Source: CAD feature listing. Evaluate the final solid. Frame: model axes, mm. Face numbers are marked on the shaded views. A direction names the side the tool comes from. Coordinates: 2 decimals unless noted, no trailing zeros. Order: outer loops, then holes, each group sorted by start corner. A loop starts at its lowest first (then second) coordinate and runs counter-clockwise, first axis right, second up.
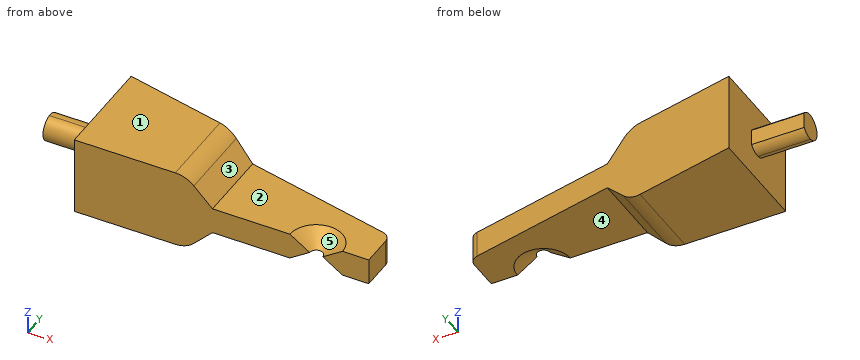
Autodesk Inventor part; units mm, degrees
ref_plane "Work Plane2" through (15.7073, 3, 0) normal (-1, 0, 0) x (0, 0, -1)
ref_plane "Work Plane5" through (10.5053, 0, 0) normal (0, 0, 1) x (1, 0, 0)
ref_plane "YZ Plane" through (0, 0, 0) normal (1, 0, 0) x (0, 1, 0)
sketch "Sketch1" plane through (0, 0, 0) normal (0, 0, 1) x (1, 0, 0)
  line L0 (0, 8) -> (22.3923, 3)
  line L1 (22.3923, 0) -> (22.3923, 3)
  line L2 (0, 0) -> (22.3923, 0)
  line L3 (0, 8) -> (0, 0)
  dimension "d5" = 3
  dimension "d7" = 8
  dimension "d59" = 22.3923
extrude "Extrusion1" add sketch "Sketch1" along normal mid plane 6
sketch "Sketch2" plane through (0, 0, 3) normal (-1, 0, 0) x (0, 0, 1)
  line L0 (-6, 0) -> (-6, 8)
  line L1 (0, 3) -> (0, 8)
  line L2 (-6, 0) -> (0, 8)
  line L3 (-6, 8) -> (0, 8)
  line L4 (0, 8) -> (0, 0)
  line L5 (-6, 8) -> (0, 0)
  arc A0 (-3.995, 3.9001) -> (-2.005, 3.9001) centre (-3, 4) ccw
  line L6 (-3.6, 4.8) -> (-2.4, 4.8)
  arc A1 (-2.005, 3.9001) -> (-2.4, 4.8) centre (-3, 4) ccw
  arc A2 (-3.6, 4.8) -> (-3.9949, 3.8993) centre (-3, 4) ccw
  point P0 (-3, 0)
extrude "Extrusion2" add sketch "Sketch2" along normal blind 4 contours A0 A2 L5 L2 | L2 L5 A0 | L6 L2 L5 | L2 A1 A0 L5
sketch "Sketch3" plane through (0, 0, 3) normal (0, -1, 0) x (1, 0, 0)
  line L0 (22.3923, -6) -> (0, -6)
  line L1 (8.5053, -6) -> (10.5053, -4)
  line L2 (10.5053, -4) -> (22.3923, -4)
  line L3 (22.3923, 0) -> (22.3923, -6)
  line L4 (22.3923, -4) -> (22.3923, -6)
  line L5 (22.3923, -6) -> (8.5053, -6)
  line L6 (8.5053, 0) -> (10.5053, -2)
  line L7 (10.5053, -2) -> (22.3923, -2)
  line L8 (22.3923, -2) -> (22.3923, 5.9236)
  line L9 (22.3923, 0) -> (0, 0)
  line L10 (8.5053, 0) -> (22.3923, 0)
  point P0 (0, -3)
  dimension "d13" = 2
  dimension "d14" = 2
  dimension "d15" = 45
extrude "Extrusion3" cut sketch "Sketch3" against normal through all
ref_plane "Work Plane2" through (15.7073, 3, 0) normal (-1, 0, 0) x (0, 0, -1)
ref_plane "Work Plane1" through (22.3923, 3, 0) normal (-1, 0, 0) x (0, 0, -1)
fillet "Fillet8" radius 2 1 edges at (8.5053, 3.0504, 3)
fillet "Fillet9" radius 2 1 edges at (8.5053, 3.0504, -3)
fillet "Fillet11" radius 0.8 1 edges at (22.3923, 3, 0)
sketch "Sketch13" plane through (10.5053, 0, 1) normal (0, 0, 1) x (1, 0, 0)
  line L0 (0, 0) -> (11.887, 0)
  arc A0 (9.887, 0) -> (5.887, 0) centre (7.887, 0) ccw
  point P0 (-10.5053, 0)
  dimension "d86" = 4
  dimension "d88" = 4
ref_plane "Work Plane5" through (10.5053, 0, 0) normal (0, 0, 1) x (1, 0, 0)
sketch "Sketch14" plane through (10.5053, 0, 0) normal (0, 0, 1) x (1, 0, 0)
  line L0 (0, 0) -> (11.887, 0)
  arc A0 (8.387, 0) -> (7.387, 0) centre (7.887, 0) ccw
  point P0 (-10.5053, 0)
  dimension "d89" = 4
  dimension "d90" = 1
loft "Loft1" cut profiles "Sketch13", "Sketch14"
sketch "Sketch16" plane through (22.3923, 0, -1) normal (0, 0, -1) x (-1, 0, 0)
  arc A0 (6, 0) -> (2, 0) centre (4, 0) ccw
  line L0 (0, 0) -> (2, 0)
  line L1 (6, 0) -> (11.887, 0)
  line L2 (2, 0) -> (6, 0)
  line L3 (11.887, 0) -> (0, 0)
  point P0 (22.3923, 0)
  dimension "d98" = 4
  dimension "d99" = 4
sketch "Sketch17" plane through (10.5053, 0, 0) normal (0, 0, 1) x (1, 0, 0)
  line L0 (11.887, 2.3589) -> (11.887, 0)
  line L1 (9.887, 0) -> (8.387, 0)
  line L2 (8.8124, 0) -> (7.1201, 0)
  arc A0 (8.387, 0) -> (7.387, 0) centre (7.887, 0) ccw
  point P0 (-10.5053, 0)
  dimension "d102" = 4
  dimension "d103" = 1
loft "Loft2" cut profiles "Sketch16" section 2 edges at (18.3923, 0.5, 0) (18.3923, 0, 0)
properties part number "blade" material "Stainless Steel"
Q1. Section query A-A on z = 0.25. Output: boundary loops of the cut face in (x, y) (3 decimals).
Solutions:
outline: (-4, 3.032) - (0, 3.032) - (0, 0) - (17.517, 0) arc R0.875 cw to (19.267, 0) - (22.392, 0) - (22.392, 2.359) arc R0.8 ccw to (21.767, 3.14) - (0, 8) - (0, 4.8) - (-4, 4.8) - close
Q2. Pin query (flat end, axial travel): P1, Ø2, axis at y = 6, z = 0, coming from the -X side; P2, Ø1.7, axis at x = 14.5, y = 3, coming from the -Z side; P3, Ø3, axis at x = 16, y = 3, coming from the +Z side. Return the tip coordinate at first contact, or that it passes through.
Solutions:
P1: stops at x = 0
P2: stops at z = -1
P3: stops at z = 1
Q3. Set-up query: the marked faces 1 and 2. Return all of +Z, -Z, +X, -X, +Y, -Y with unobstructed straight access to the full face (end or side cutting, diameter ignored); none if empty.
Solutions:
face 1: +Z, +X, -X, +Y, -Y
face 2: +Z, +X, +Y, -Y
Q4. Pull-direction query (X, two-part tool) for the marked faces 3, 4 and 5; classes: pulls with the +X half, pulls with the -X half, needs draft (parallel to the pull), parting line crosses it, or undercut.
Solutions:
face 3: pulls with the +X half
face 4: needs draft
face 5: undercut
Q5. Material intervals for line 1 along Z through (x, y) = (21, 1.5); line 2 along Z through (x, y) = (7.75, 3.75); line 3 along X through (y, z) = (5, -1.75), sorted ascending.
Solutions:
line 1: z = -1 to 1
line 2: z = -3 to 3
line 3: x = 0 to 9.76
Q6. Section query C-C on y = 7.25. Output: boundary loops of the cut face in (x, z), plus the area to 3 significant figures.
Solutions:
outline: (0, -3) - (3.36, -3) - (3.36, 3) - (0, 3) - close
area: 20.2 mm2
Q7. Section query B-B on x = 1. Output: boundary loops of the cut face in (y, z), plus the area to 3 significant figures.
Solutions:
outline: (0, -3) - (7.78, -3) - (7.78, 3) - (0, 3) - close
area: 46.7 mm2
